Geometry: final body of the model. Coordinates: model frame, mm. A direction names the side the tool comes from. Round coordinates to 2 decimals unless told otherwise and drop trailing zeros. Write each loop counter-clockwise with the first axis right and the second up, starting at its lowest first coordinate (ties: lowest second). Pieces come first, ordered by that corner, then holes. Notation, with made-up numbers: (12, 9.5) -> (34, 9.5) arc R38 ccw to (34, 48.5) -> close; hole circle Ø8 at (59.25, -37). An arc over 180 degrees is marked (long way). One line per item, written item: value. Start each with the question number.
Autodesk Inventor part; units mm, degrees
ref_plane "Plano inicial" through (0, 0, -18.3012) normal (0, 0, 1) x (1, 0, 0)
ref_plane "Plano final" through (0, 0, 648.3012) normal (0, 0, 1) x (1, 0, 0)
ref_plane "Plano de trabajo4" through (0, 20, -20) normal (0, -0.7071, -0.7071) x (1, 0, 0)
ref_plane "Plano inicial" through (0, 0, -18.3012) normal (0, 0, 1) x (1, 0, 0)
ref_plane "Plano final" through (0, 0, 648.3012) normal (0, 0, 1) x (1, 0, 0)
sketch "Boceto" plane through (0, 0, 0) normal (0, 0, 1) x (1, 0, 0)
  line L0 (-14.2, 20) -> (14.2, 20)
  line L1 (20, 14.2) -> (20, -14.2)
  line L2 (14.2, -20) -> (-14.2, -20)
  line L3 (-20, -14.2) -> (-20, 14.2)
  arc A0 (-14.2, 20) -> (-20, 14.2) centre (-14.2, 14.2) ccw
  arc A1 (20, 14.2) -> (14.2, 20) centre (14.2, 14.2) ccw
  arc A2 (14.2, -20) -> (20, -14.2) centre (14.2, -14.2) ccw
  arc A3 (-20, -14.2) -> (-14.2, -20) centre (-14.2, -14.2) ccw
  line L4 (-29.6817, 0) -> (29.6817, 0) construction
  line L5 (0, -29.6817) -> (0, 29.6817) construction
  arc A4 (-14.2, 17.1) -> (-17.1, 14.2) centre (-14.2, 14.2) ccw
  line L6 (-14.2, 17.1) -> (14.2, 17.1)
  arc A5 (17.1, 14.2) -> (14.2, 17.1) centre (14.2, 14.2) ccw
  line L7 (17.1, 14.2) -> (17.1, -14.2)
  arc A6 (14.2, -17.1) -> (17.1, -14.2) centre (14.2, -14.2) ccw
  line L8 (14.2, -17.1) -> (-14.2, -17.1)
  arc A7 (-17.1, -14.2) -> (-14.2, -17.1) centre (-14.2, -14.2) ccw
  line L9 (-17.1, -14.2) -> (-17.1, 14.2)
  point P0 (-20, 20)
  point P1 (20, -20)
  point P2 (20, 20)
  dimension "b" = 40
  dimension "msp_r" = 5.8
  dimension "d8" = 20
  dimension "d9" = 20
  dimension "d10" = 2.9
extrude "Cuerpo" add sketch "Boceto" along normal up to surface (666.6024 mm away) from surface at -18.3012
sketch "Sketch2" plane through (0, 0, 0) normal (0, 0, 1) x (1, 0, 0)
  line L0 (0, 0) -> (10, 0)
ref_plane "Work Plane3" through (0, 0, 0) normal (0, -1, 0) x (1, 0, 0)
sketch "Sketch3" plane through (0, 0, 0) normal (0, -1, 0) x (1, 0, 0)
  line L0 (-2, -18.3012) -> (12, -18.3012)
  line L1 (-2, 648.3012) -> (12, 648.3012)
  dimension "d14" = 666.6024
ref_plane "Plano de trabajo4" through (0, 20, -20) normal (0, -0.7071, -0.7071) x (1, 0, 0)
split "Dividir1" plane through (0, 20, -20) removes the side toward (0, -0.7071, -0.7071)
ref_plane "Plano de trabajo5" through (-20, 0, -20) normal (0.7071, 0, -0.7071) x (-0.7071, 0, -0.7071)
split "Dividir2" plane through (-20, 0, -20) removes the side toward (0.7071, 0, -0.7071)
ref_plane "Plano de trabajo6" through (-20, 0, 650) normal (0.7071, 0, 0.7071) x (0.7071, 0, -0.7071)
split "Dividir3" plane through (-20, 0, 650) removes the side toward (0.7071, 0, 0.7071)
ref_plane "Plano de trabajo7" through (0, 20, 650) normal (0, -0.7071, 0.7071) x (1, 0, 0)
split "Dividir4" plane through (0, 20, 650) removes the side toward (0, -0.7071, 0.7071)
equation "\"msp_r\" = 2 * ParT"
equation "\"d8\" = d9"
equation "\"d9\" = 0.5 * b"
equation "\"d10\" = ParT"
equation "\"G_OFFSET_START\" = 18.30122"
equation "\"G_OFFSET_END\" = 18.30122"
equation "\"d11\" = -G_OFFSET_START"
equation "\"d12\" = G_OFFSET_END + B_L"
equation "\"G_L\" = d14"
properties part number "DIN 59 410 - 40x40x2.9-666.602" material "Acero, suave"
(1) Section query C-C (z = 564.5). Output: boundary loops of the cut face in (x, y), and give its area (3 significant figures).
(2) Line query: probe 1 along Y at (x, z) = (-14, 512); probe 2 along Y at (x, z) = (-7, 11.5). Output: solid intervals per line, ascending.
(3) Section query B-B (x = 4.5). Output: boundary loops of the cut face in (y, z), and give its area (3 significant figures).
(4) Section query A-A (y = 5). Output: boundary loops of the cut face in (x, z), and give its area (3 significant figures).
(5) Pull-direction query (X, two-part tool) for faces 1 (the face through (-20, 0, 310)), 2 (the face through (0, -17.1, 311)), 3 (the face through (9, 18, 9)); classes: pulls with the +X half, pulls with the -X half, needs draft (parallel to the pull), parting line crosses it, or undercut.
(6) Set-up query: faces 4 (the face through (0, 17.1, 310)), 5 (the face through (0, -20, 311)). Return all of +Z, -Z, +X, -X, +Y, -Y with unobstructed straight access to the full face (end or side cutting, diameter ignored); none if empty.
Results list:
1. outline: (-20, -14.2) arc R5.8 ccw to (-14.2, -20) -> (14.2, -20) arc R5.8 ccw to (20, -14.2) -> (20, 14.2) arc R5.8 ccw to (14.2, 20) -> (-14.2, 20) arc R5.8 ccw to (-20, 14.2) -> close; hole (-17.1, -14.2) arc R2.9 ccw to (-14.2, -17.1) -> (14.2, -17.1) arc R2.9 ccw to (17.1, -14.2) -> (17.1, 14.2) arc R2.9 ccw to (14.2, 17.1) -> (-14.2, 17.1) arc R2.9 ccw to (-17.1, 14.2) -> close
1. area: 409 mm^2
2. probe 1: y = -20 to -17.1, 17.1 to 20
2. probe 2: y = 17.1 to 20
3. outline: (-20, 20) -> (-17.1, 17.1) -> (-17.1, 612.9) -> (-20, 610) -> close; (17.1, 4.5) -> (20, 4.5) -> (20, 625.5) -> (17.1, 625.5) -> close
3. area: 3,520 mm^2
4. outline: (-20, -5) -> (-17.1, -5) -> (-17.1, 635) -> (-20, 635) -> close; (17.1, 17.1) -> (20, 20) -> (20, 610) -> (17.1, 612.9) -> close
4. area: 3,580 mm^2
5. face 1: pulls with the -X half
5. face 2: undercut
5. face 3: pulls with the +X half
6. face 4: +Z, -Z
6. face 5: +Z, -Z, +X, -X, -Y
